```python
from build123d import *

# Parameters (mm, degrees)
F0_R     = 2.554654
F0_R_2   = 1.573486
F0_R_3   = 3
F1_DEPTH = 10


with BuildPart() as f1:
    # F0 (on Front) → F1 (new body)
    with BuildSketch(Plane.XZ):
        Polygon((-57.889797, 80.625616), (-57.889797, 1.519148), (-30.889797, 1.519148), (-30.889797, 112.519148), align=None)
        with Locations((-51.889797, 7.519148)):
            Circle(F0_R, mode=Mode.SUBTRACT)
        with Locations((-39.247134, 11.526519)):
            Circle(F0_R_2, mode=Mode.SUBTRACT)
        with Locations((-51.889797, 77.519148)):
            Circle(F0_R_3, mode=Mode.SUBTRACT)
        with Locations((-39.247134, 81.3893)):
            Circle(F0_R_2, mode=Mode.SUBTRACT)
    extrude(amount=-F1_DEPTH)


solid = f1.part
```
Source: CAD feature listing. Evaluate the final solid. Frame: model axes, mm. Give positions to 0.01 mm unless a question says otherwise; leave off trailing zeros. Loops run counter-clockwise (first coordinate to the right, second up) from the corner with the lowest first, then second, coordinate; pieces in that order, holes last. Notation, with made-up numbers: (-22.5, 51.25) -> (13.5, 51.25) arc R28 ccw to (13.5, 84.25) -> close; hole circle Ø1 at (-23, 17). An arc over 180 degrees is marked (long way). Use a Markdown table: item, result. Add a question column.
(1) Section query D-D (x = -35.5). Output: boundary loops of the cut face in (y, z).
(2) First-contact query: pin 1 Ø3 at (x, z) = (-51.5, 83.5) entering from -Y; pin 2 Ø4.5 at (x, z) = (-51.89, 7.52) entering from +Y. Flat tips, straight axial feed; report the tip coordinate or a pass-through.
(3) Ray query, line 1 (Z direction, x = -51, y = 9); line 2 (Z direction, x = -40, y = 6.25); line 3 (Z direction, x = -49.25, y = 7.5). Return the intervals inside material, ascending.
(4) Section query A-A (x = -53.5). Output: boundary loops of the cut face in (y, z).
(5) Pull-direction query (Z, two-part tool) for faces 1 (the face through (-49.453, 4.93, 8.286)), 2 (the face through (-40.4, 4.9, 12.6)), 3 (the face through (-45, 5, 1.519)), 4 (the face through (-30.89, 5, 56)); classes: +Z half, -Z half, draft (parallel to the pull), parting line (faces both ways), or undercut.
(6) Section query C-C (z = 100.5). Output: boundary loops of the cut face in (x, y), then the cut area to 3 significant figures.
(7) Section query B-B (y = 3.5). Output: boundary loops of the cut face in (x, z), then the cut area to 3 significant figures.
Checked values:
| question | item | result |
|---|---|---|
| 1 | outline | (0, 1.52) -> (10, 1.52) -> (10, 107.07) -> (0, 107.07) -> close |
| 2 | pin 1 | y = 0 |
| 2 | pin 2 | through |
| 3 | line 1 | 1.52 to 5.12, 9.91 to 74.65, 80.38 to 88.76 |
| 3 | line 2 | 1.52 to 10.14, 12.91 to 80.01, 82.77 to 101.76 |
| 3 | line 3 | 1.52 to 76.09, 78.94 to 90.83 |
| 4 | outline | (0, 1.52) -> (10, 1.52) -> (10, 5.54) -> (0, 5.54) -> close; (0, 9.5) -> (10, 9.5) -> (10, 74.99) -> (0, 74.99) -> close; (0, 80.05) -> (10, 80.05) -> (10, 85.81) -> (0, 85.81) -> close |
| 5 | face 1 | undercut |
| 5 | face 2 | undercut |
| 5 | face 3 | -Z half |
| 5 | face 4 | draft |
| 6 | outline | (-41.06, 0) -> (-30.89, 0) -> (-30.89, 10) -> (-41.06, 10) -> close |
| 6 | area | 102 mm^2 |
| 7 | outline | (-57.89, 1.52) -> (-30.89, 1.52) -> (-30.89, 112.52) -> (-57.89, 80.63) -> close; hole circle Ø6 at (-51.89, 77.52); hole circle Ø5.11 at (-51.89, 7.52); hole circle Ø3.15 at (-39.25, 11.53); hole circle Ø3.15 at (-39.25, 81.39) |
| 7 | area | 2,500 mm^2 |
